from build123d import *

# Parameters (mm, degrees)
F0_W     = 43.18
F0_H     = 17.272
F2_DEPTH = 76.2
F3_DEPTH = 69.85
F6_ANGLE = 45
F8_W     = 97.1712954342
F8_H     = 80.9760764241
F8_W_2   = 68.9119933241
F8_H_2   = 39.37
F9_DEPTH = 38.1
F10_R    = 0.762


# Not quite as in the source:
# - ends of sketch curves that miss each other by under 0.0002 mm in the source are joined


with BuildPart() as f2:
    # F0 (on Front) → F2 (new body)
    with BuildSketch(Plane.XZ):
        Rectangle(F0_W, F0_H)
    extrude(amount=-F2_DEPTH)

    # F1 (on Front) → F3 (cut)
    with BuildSketch(Plane.XZ):
        with BuildLine():
            Line((10.1640512741, -1.0311319662), (10.1640512741, 1.5088680338))
            Line((10.1640512741, 1.5088680338), (19.304, 3.81))
            Line((19.304, 3.81), (19.304, 7.874))
            Line((19.304, 7.874), (10.1640512741, 4.0488680338))
            ThreePointArc((10.1640512741, 4.0488680338), (7.567989059, 4.950925683), (4.8339106143, 4.6715297537))
            Line((4.8339106143, 4.6715297537), (1.97346e-05, 4.6852644338))
            Line((1.97346e-05, 4.6852644338), (-4.8339106143, 4.6715297537))
            ThreePointArc((-4.8339106143, 4.6715297537), (-7.567989059, 4.950925683), (-10.1640512741, 4.0488680338))
            Line((-10.1640512741, 4.0488680338), (-19.304, 7.874))
            Line((-19.304, 7.874), (-19.304, 3.81))
            Line((-19.304, 3.81), (-10.1640512741, 1.5088680338))
            Line((-10.1640512741, 1.5088680338), (-10.1640512741, -1.0311319662))
            Line((-10.1640512741, -1.0311319662), (-19.304, -3.81))
            Line((-19.304, -3.81), (-19.304, -7.874))
            Line((-19.304, -7.874), (-10.1640512741, -3.81))
            Line((-10.1640512741, -3.81), (-1.778, -3.81))
            Line((-1.778, -3.81), (-1.778, -7.874))
            Line((-1.778, -7.874), (-1.778, -8.9796995744))
            Line((-1.778, -8.9796995744), (1.778, -8.9796995744))
            Line((1.778, -8.9796995744), (1.778, -7.874))
            Line((1.778, -7.874), (1.778, -3.81))
            Line((1.778, -3.81), (10.1640512741, -3.81))
            Line((10.1640512741, -3.81), (19.304, -7.874))
            Line((19.304, -7.874), (19.304, -3.81))
            Line((19.304, -3.81), (10.1640512741, -1.0311319662))
        make_face()
    extrude(amount=-F3_DEPTH, mode=Mode.SUBTRACT)


with BuildPart() as f2_1:
    # F4: moved
    add(f2.part.moved(Location((0, -38.1, 0))))


with BuildPart() as f2_2:
    # F6: moved
    add(f2_1.part.rotate(Axis((-4.1610468179, 0, 0), (-1, 0, 0)), F6_ANGLE))

    # F8 (on Right) → F9 (cut, symmetric)
    with BuildSketch(Plane.YZ):
        with Locations((-6.1953347176, -4.1167326272)):
            Rectangle(F8_W, F8_H)
        with Locations((-5.4169551435, -9.6378130603)):
            Rectangle(F8_W_2, F8_H_2, mode=Mode.SUBTRACT)
    extrude(amount=F9_DEPTH, both=True, mode=Mode.SUBTRACT)

    # F10
    f10_edges = [f2_2.edges().sort_by_distance(p)[0] for p in [
        (21.59, 20.834194, -29.322813),
        (-21.59, 20.834194, -29.322813),
    ]]
    fillet(f10_edges, radius=F10_R)


solid = f2_2.part
Input: part model. Units: mm. Frame: model coordinates. A direction names the side the tool comes from. Round coordinates to 2 decimals unless told otherwise and drop trailing zeros. Order: outer loops, then holes, each group sorted by start corner. A loop starts at its lowest first (then second) coordinate and runs counter-clockwise, first axis right, second up. Notation, with made-up numbers: (-12, 18) - (19, 18) arc R22 cw to (19, 25) - close; hole circle Ø2 at (-12.5, -21.75). An arc over 180 degrees is marked (long way). Answer as a JSON object with one key per item and string values. Group by question number.
(1) Cut plane B-B (z = -24). Return loops of the section in (x, y).
(2) Reachability of faces 1 (the face through (-19.304, 11, -3)), 2 (the face through (0, 29.039, -21)) from +Z, -Z, +X, -X, +Y, -Y: full face, straight path, thin tool, end or side. Return the list, or none.
(3) Cut plane D-D (y = -1.5). Count the separate pieces of the cut face and the enclosed holes in it, then the cut area to 3 significant figures.
(4) Cut plane C-C (x = -3.5). Return loops of the section in (y, z).
(5) Draft query along X for faces 3 (the face through (-0.3, 26.83, -27.05)), 4 (the face through (14.8, 2.88, -6.33)). Return one class per face: released by +X, released by -X, zero draft, split by the parting line, or undercut.
(6) Material intervals for probe 1 along Y at (x, z) = (-12, -10.5); probe 2 along Y at (x, z) = (-12, -14.5); probe 3 along X at (y, z) = (18, -24.5), sorted ascending. Write a range as from..to.
(7) Pin query (flat end, axial travel): P1, Ø5, axis at x = 5, z = 0.5, coming from the -Y side; P2, Ø6, axis at x = 10, y = 7.5, coming from the -Z side; P3, Ø6, axis at x = -13.5, y = -6, coming from the -Z side. Return the tip coordinate at first contact, or that it passes through.
(8) Cut plane A-A (y = -9.5). Return loops of the section in (x, z), then the cut area to 3 significant figures.
Here are the results:
{
 "1": {"outline": "(-21.59, 11.79) - (-1.78, 11.79) - (-1.78, 18.61) - (-10.16, 18.61) - (-19.3, 12.86) - (-19.3, 18.61) - (-13.98, 20.9) - (13.98, 20.9) - (19.3, 18.61) - (19.3, 12.86) - (10.16, 18.61) - (1.78, 18.61) - (1.78, 11.79) - (21.59, 11.79) - (21.59, 29.04) - (-21.59, 29.04) - close"},
 "2": {"face 1": "none", "face 2": "+Z, -Z, +X, -X, +Y"},
 "3": {"separate pieces": "3", "enclosed holes": "0", "area": "464 mm^2"},
 "4": {"outline": "(-22.26, 10.05) - (17.11, -29.32) - (24.56, -29.32) - (29.04, -24.84) - (29.04, -16.83) - (2.17, 10.05) - (-3.44, 10.05) - (25.76, -19.14) - (19.76, -25.14) - (-15.44, 10.05) - close"},
 "5": {"face 3": "zero draft", "face 4": "undercut"},
 "6": {"probe 1": "y = -1.71..3.96, 8.25..13.29, 17.31..22.71", "probe 2": "y = 2.29..7.96, 12.25..17.29, 21.31..26.71", "probe 3": "x = -21.59..-19.3, -11.93..-1.78, 1.78..11.93, 19.3..21.59"},
 "7": {"P1": "stops at y = -15.21", "P2": "stops at z = -22.71", "P3": "stops at z = -9.21"},
 "8": {"outline": "(-21.59, -2.71) - (-1.78, -2.71) - (-1.78, 4.11) - (-10.16, 4.11) - (-19.3, -1.64) - (-19.3, 4.11) - (-10.16, 8.04) - (-10.16, 10.05) - (-21.59, 10.05) - close; (1.78, -2.71) - (21.59, -2.71) - (21.59, 10.05) - (10.16, 10.05) - (10.16, 8.04) - (19.3, 4.11) - (19.3, -1.64) - (10.16, 4.11) - (1.78, 4.11) - close", "area": "318 mm^2"}
}
